CAD build for the part. Positions are in the model's coordinates, mm. Face numbers are marked on the shaded views. Coordinates: 2 decimals unless noted, no trailing zeros. Write each loop counter-clockwise with the first axis right and the second up, starting at its lowest first coordinate (ties: lowest second). Pieces come first, ordered by that corner, then holes. Notation, with made-up numbers: (-8.75, 32.25) - (37.25, 32.25) arc R14 cw to (37.25, 46.25) - close; hole circle Ø7 at (38.25, -2.75). An arc over 180 degrees is marked (long way). Answer in a Markdown table with one row per item. Add a question column.
Q1. Band-saw the part on D-D (x = 31). List the corners of the cut face in (y, z), and give its area (3 significant figures).
Q2. Drill centre lines: line 1 along X through (y, z) = (6.5, -265); line 2 along Z through (x, y) = (71, 12); line 3 along X through (y, z) = (12.75, -40). Where is each one in solid material? Low to high. Write a range as from..to.
Q3. Two-plate mould, pull along X, no slides. Class the marked faces 1 and 2: +X half, -X half, draft (parallel to the pull), parting line (faces both ways), or undercut.
Q4. Band-saw the part on A-A (z = -265). List the corners of the cut face in (x, y), and give its area (3 significant figures).
Q5. Pin check, flat tip, straight feed: pin 1 (1 mm diameter, centred on x = 69.5, y = 7, fed in from +Z). Stop position of the tip, or through.
Q6. Band-saw the part on C-C (x = 71). List the corners of the cut face in (y, z).
Q7. Band-saw the part on B-B (y = 22.25). List the corners of the cut face in (x, z), and give its area (3 significant figures).
```python
from build123d import *

# Parameters (mm, degrees)
SKETCH2_W           = 101.6
SKETCH2_H           = 280
BOSS_EXTRUDE1_DEPTH = 25.4
SKETCH3_R           = 6.75
CUT_EXTRUDE1_DEPTH  = 25.4
SKETCH4_R           = 16
CUT_EXTRUDE2_DEPTH  = 25.4


with BuildPart() as part:
    # Sketch2 → Boss-Extrude1 (new body)
    with BuildSketch(Plane(origin=(0, 0, 0), x_dir=(1, 0, 0), z_dir=(0, 1, 0))):
        with Locations((50.8, 140)):
            Rectangle(SKETCH2_W, SKETCH2_H)
    extrude(amount=BOSS_EXTRUDE1_DEPTH)

    # Sketch3 → Cut-Extrude1 (cut)
    with BuildSketch(Plane(origin=(0, 25.4, 0), x_dir=(1, 0, 0), z_dir=(0, 1, 0))):
        with Locations((71, 265)):
            Circle(SKETCH3_R)
        with Locations((31, 265)):
            Circle(SKETCH3_R)
        with Locations((31, 185)):
            Circle(SKETCH3_R)
        with Locations((71, 185)):
            Circle(SKETCH3_R)
    extrude(amount=-CUT_EXTRUDE1_DEPTH, mode=Mode.SUBTRACT)

    # Sketch4 → Cut-Extrude2 (cut)
    with BuildSketch(Plane(origin=(0, 25.4, 0), x_dir=(1, 0, 0), z_dir=(0, 1, 0))):
        with Locations((40, 40)):
            Circle(SKETCH4_R)
    extrude(amount=-CUT_EXTRUDE2_DEPTH, mode=Mode.SUBTRACT)


solid = part.part
```
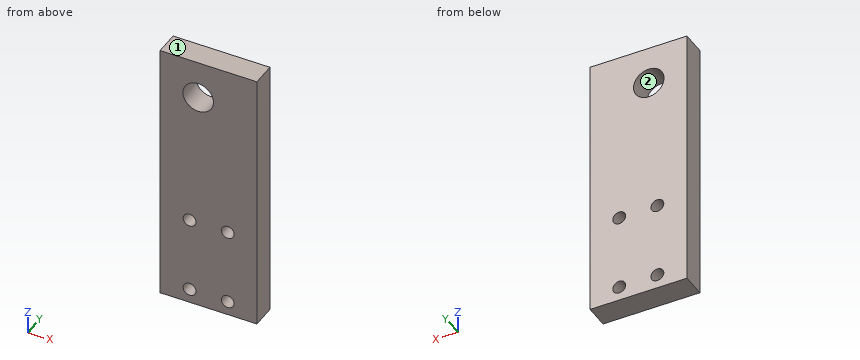
Checked values:
| question | item | result |
|---|---|---|
| 1 | outline | (0, -280) - (25.4, -280) - (25.4, -271.75) - (0, -271.75) - close; (0, -258.25) - (25.4, -258.25) - (25.4, -191.75) - (0, -191.75) - close; (0, -178.25) - (25.4, -178.25) - (25.4, -53.23) - (0, -53.23) - close; (0, -26.77) - (25.4, -26.77) - (25.4, 0) - (0, 0) - close |
| 1 | area | 5,750 mm² |
| 2 | line 1 | x = 0..24.25, 37.75..64.25, 77.75..101.6 |
| 2 | line 2 | z = -280..-271.75, -258.25..-191.75, -178.25..0 |
| 2 | line 3 | x = 0..24, 56..101.6 |
| 3 | face 1 | draft |
| 3 | face 2 | undercut |
| 4 | outline | (0, 0) - (24.25, 0) - (24.25, 25.4) - (0, 25.4) - close; (37.75, 0) - (64.25, 0) - (64.25, 25.4) - (37.75, 25.4) - close; (77.75, 0) - (101.6, 0) - (101.6, 25.4) - (77.75, 25.4) - close |
| 4 | area | 1,890 mm² |
| 5 | pin 1 | stops at z = 0 |
| 6 | outline | (0, -280) - (25.4, -280) - (25.4, -271.75) - (0, -271.75) - close; (0, -258.25) - (25.4, -258.25) - (25.4, -191.75) - (0, -191.75) - close; (0, -178.25) - (25.4, -178.25) - (25.4, 0) - (0, 0) - close |
| 7 | outline | (0, -280) - (101.6, -280) - (101.6, 0) - (0, 0) - close; hole circle Ø32 at (40, -40); hole circle Ø13.5 at (31, -265); hole circle Ø13.5 at (31, -185); hole circle Ø13.5 at (71, -265); hole circle Ø13.5 at (71, -185) |
| 7 | area | 27,100 mm² |
